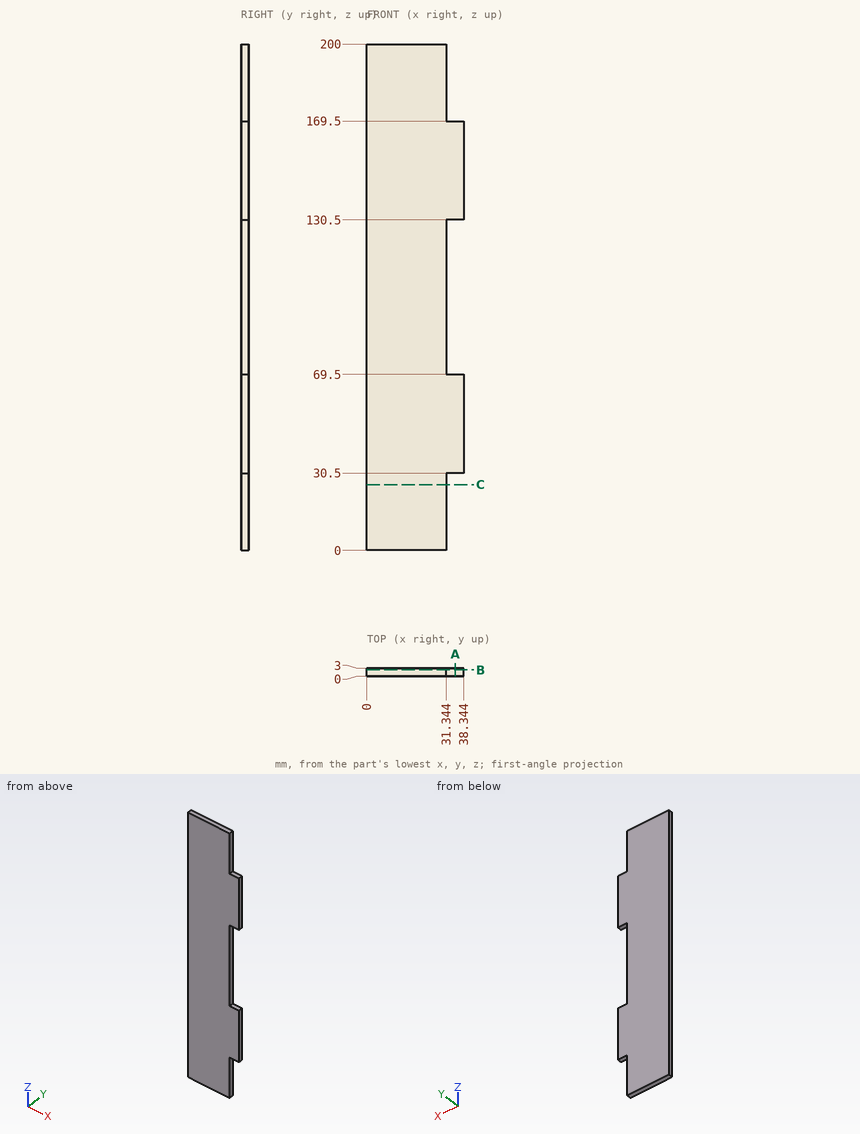
The figure shows three views and two pictorial views of one solid part (mm, origin at its lowest corner). Answer the questions. Coordinates: 2 decimals unless noted, no trailing zeros. Loops run counter-clockwise (first coordinate to the right, second up) from the corner with the lowest first, then second, coordinate; pieces in that order, holes last. Notation, with made-up numbers: (33, -38.5) - (62, -38.5) arc R8 cw to (62, -27.5) - close; hole circle Ø7 at (25, -32). An arc over 180 degrees is marked (long way). Write item = value, one per line.
1) Section B-B (y = 2.4) is taken. Determine the outline of the cut face in (x, z), plus the area to 3 significant figures.
Responses:
outline = (0, 0) - (31.34, 0) - (31.34, 30.5) - (38.34, 30.5) - (38.34, 69.5) - (31.34, 69.5) - (31.34, 130.5) - (38.34, 130.5) - (38.34, 169.5) - (31.34, 169.5) - (31.34, 200) - (0, 200) - close
area = 6,810 mm^2
2) Section C-C (z = 26) is taken. Determine the outline of the cut face in (x, y).
Responses:
outline = (0, 0) - (31.34, 0) - (31.34, 3) - (0, 3) - close
3) Find the intervals of material crossed by line 1 along Z through (x, y) = (32, 2); line 2 along X through (y, z) = (2.45, 124.5), in increasing order.
Responses:
line_1 = 30.5 to 69.5, 130.5 to 169.5
line_2 = 0 to 31.34
4) Each of these flat-tipped pins is pushed along its axis until it touches: P1, Ø0.9, axis at y = 1.5, z = 190, coming from the +X side; P2, Ø0.9, axis at x = 35, y = 1, coming from the +Z side. Where does it stop, or does it pass through?
Responses:
P1 = 31.34
P2 = 169.5
5) Section A-A (x = 35) is taken. Determine the outline of the cut face in (y, z).
Responses:
outline = (0, 30.5) - (3, 30.5) - (3, 69.5) - (0, 69.5) - close; (0, 130.5) - (3, 130.5) - (3, 169.5) - (0, 169.5) - close
